Here's how the part is built. I have some questions about the finished solid (model axes, mm). Round coordinates to 2 decimals unless told otherwise and drop trailing zeros. Loops run counter-clockwise (first coordinate to the right, second up) from the corner with the lowest first, then second, coordinate; pieces in that order, holes last. Notation, with made-up numbers: M 38.25,81.25 L 57.25,81.25 A13 ccw 57.25,91.25 Z; hole C -14.5,87.25 d5. An arc over 180 degrees is marked long. Use a Markdown table: item, result.
```python
from build123d import *

# Parameters (mm, degrees)
CUT_EXTRUDE1_START = -25.4
SKETCH2_W          = 6.35
SKETCH2_H          = 19.05
CUT_EXTRUDE1_DEPTH = 25.4


with BuildPart() as part:
    # Sketch1 → Revolve1 (revolve)
    with BuildSketch(Plane.XY):
        Polygon((520.646295907, -1547.882062127), (519.936476988, -1549.372685521), (315.784745775, -1452.157814294), (316.494564694, -1450.6671909), align=None)
    revolve(axis=Axis((319.879854926, -1443.558063946, 0), (0.902860929, -0.429932719, 0)))

    # Sketch2 → Cut-Extrude1 (cut)
    with BuildSketch(Plane(origin=(1025.2494541, -488.212826138, 0), x_dir=(0, 0, -1), z_dir=(0.902860929, -0.429932719, 0)).offset(CUT_EXTRUDE1_START)):
        with Locations((0, -1165.805358667)):
            Rectangle(SKETCH2_W, SKETCH2_H)
    extrude(amount=CUT_EXTRUDE1_DEPTH, mode=Mode.SUBTRACT)


solid = part.part
```
Q1. I need wall thicknesses on line 1 (Y direction, x = 453, z = -0.5); line 2 (Y direction, x = 437.5, z = -2); line 3 (Z direction, x = 414, y = -1489.5). Which ranges of each line are inside material? Lowest first, please. Write a range as from..to.
Return value:
| item | result |
|---|---|
| line 1 | y = -1517.48..-1515.65, -1498.24..-1496.41 |
| line 2 | y = -1509.88..-1508, -1491.13..-1489.25 |
| line 3 | z = -9.47..-7.81, 7.81..9.47 |
Q2. Imagine slicing it at A-A, the plane z = 5.25. Please give me the cut outline in (x, y).
Return value:
| item | result |
|---|---|
| outline | M 316.46,-1450.73 L 520.61,-1547.95 L 521.51,-1546.07 L 317.36,-1448.86 Z; M 322.4,-1438.26 L 526.55,-1535.47 L 527.45,-1533.6 L 323.3,-1436.38 Z |
Q3. We'd pull the mould along Y, two halves only. Please class faces 1 (the cylindrical face through (426.767, -1485.744, -0.346)), 2 (the flat face through (524.3, -1540.21, -8.01)), 3 (the flat face through (516, -1528, 3.175)): pulls with the +Y half, pulls with the -Y half, needs draft (parallel to the pull), parting line crosses it, or undercut.
Return value:
| item | result |
|---|---|
| face 1 | undercut |
| face 2 | pulls with the -Y half |
| face 3 | needs draft |
Q4. Will these pins go through, and if not, where does the flat tip stop? P1, Ø14, axis at x = 506.5, y = -1543, coming from the +Z side; P2, Ø3, axis at x = 471.5, y = -1508.5, coming from the +Z side; P3, Ø6.5, axis at x = 504.5, y = -1539.5, coming from the -Z side.
Return value:
| item | result |
|---|---|
| P1 | stops at z = 9.18 |
| P2 | stops at z = 8.07 |
| P3 | stops at z = -8.65 |
